Autodesk Inventor part; units mm, degrees
ref_plane "YZ Plane" through (0, 0, 0) normal (1, 0, 0) x (0, 1, 0)
ref_plane "XZ Plane" through (0, 0, 0) normal (0, 1, 0) x (-1, 0, 0)
ref_plane "XY Plane" through (0, 0, 0) normal (0, 0, 1) x (1, 0, 0)
sketch "草图1" plane through (0, 0, 0) normal (0, 0, 1) x (1, 0, 0)
  circle A0 centre (0, 0) radius 9.5
  dimension "d0" = 19
extrude "拉伸1" add sketch "草图1" along normal blind 4
sketch "草图2" plane through (0, 0, 0) normal (0, 0, -1) x (-1, 0, 0)
  circle A0 centre (0, 0) radius 9.5
  circle A1 centre (0, 0) radius 7
  dimension "d3" = 14
extrude "拉伸2" add sketch "草图2" along normal blind 3 contours A1
sketch "草图3" plane through (0, 0, -3) normal (0, 0, -1) x (-1, 0, 0)
  circle A0 centre (0, 0) radius 7
  circle A1 centre (0, 0) radius 8.3315
  dimension "d6" = 14
  dimension "d7" = 16.663
extrude "拉伸3" add sketch "草图3" along normal blind 7 contours A0 | A1
thread "螺纹1"
chamfer "倒角1" distance 1 angle 45 2 edges at (8.3315, 0, -10) (-9.5, 0, 4)
sketch "草图4" plane through (0, 0, 4) normal (0, 0, 1) x (1, 0, 0)
  circle A0 centre (0, 0) radius 8.5
  line L0 (0, 0) -> (0, 1)
  line L1 (0, 1) -> (21.5358, 1)
  line L2 (21.5358, 1) -> (-22.0631, 1)
  line L3 (-22.0631, 1) -> (-22.0631, -1)
  line L4 (-22.0631, -1) -> (21.5358, -1)
  line L5 (21.5358, -1) -> (21.5358, 1)
  dimension "d15" = 1
  dimension "d16" = 2
extrude "拉伸4" cut sketch "草图4" against normal blind 2 contours A0 L4 L2 L1 | A0 L1 L5 L4 | A0 L4 L3 L2
properties part number "螺塞" material "钢 AISI 1018 106 HR"
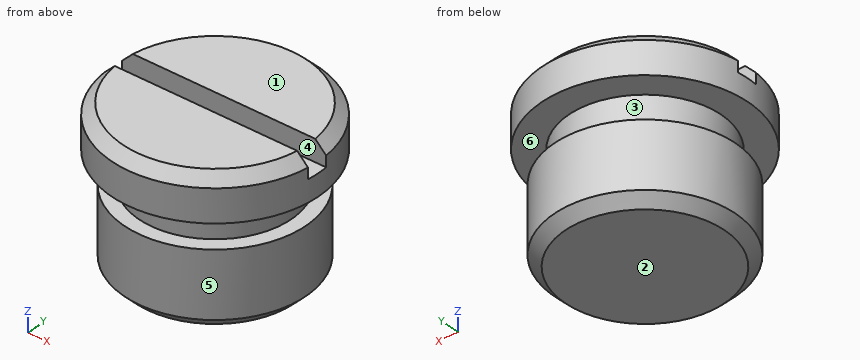
Design review of the part built by this model. Coordinates are the model's own, in mm. Face numbers are marked on the shaded views. A direction names the side the tool comes from. Give positions to 0.01 mm unless a question says otherwise; leave off trailing zeros. Loops run counter-clockwise (first coordinate to the right, second up) from the corner with the lowest first, then second, coordinate; pieces in that order, holes last. Notation, with made-up numbers: (67.5, 30) -> (121.5, 30) arc R29 cw to (121.5, 67) -> close; hole circle Ø3 at (-32.5, -11). An arc over 180 degrees is marked (long way). One line per question, with ' | ' between items. Start each with the question number.
(1) For the marked faces 4, 5 and 6, list the 3-axis set-ups (+Z, -Z, +X, -X, +Y, -Y) from which the entire face can be reached by the end or side of a thin tool; tool diameter is ignored.
(2) We need section B-B (y = 0). State the section outline as (x, z) points, and give its area (3 significant figures).
(3) We need section D-D (z = 1.25). State the section outline as (x, y) points.
(4) We need section C-C (z = -8.5). State the section outline as (x, y) points.
(5) For line 1 (Z direction, x = 0.25, y = -0.5); line 2 (Z direction, x = -3, y = -6.5); line 3 (Z direction, x = 6.75, y = 3.5), list the stretches that pass through material, from the lowest coordinate up.
(6) We need section A-A (x = 0). State the section outline as (y, z) points.
(7) Insertion check: P1, Ø2, axis at x = 4.5, z = -5.5, coming from the +Y side; P2, Ø8, axis at x = 4.5, z = -3, coming from the +Y side; P3, Ø3, axis at y = 5.5, z = -4.5, coming from the -X side. Each pin has a flat end and moves straight along its axis. Give the tip position at first contact, or say it passes through.
(8) Draft analysis for pull direction Z (two halves, no side actions). For the marked faces 1, 2 and 3, state which applies: +Z half, -Z half, draft (parallel to the pull), parting line (faces both ways), or undercut.
The answers:
1) face 4: +Z, +X, -X | face 5: -Z | face 6: none
2) outline: (-9.5, 0) -> (-7, 0) -> (-7, -3) -> (-8.33, -3) -> (-8.33, -9) -> (-7.33, -10) -> (7.33, -10) -> (8.33, -9) -> (8.33, -3) -> (7, -3) -> (7, 0) -> (9.5, 0) -> (9.5, 2) -> (-9.5, 2) -> close | area: 196 mm^2
3) outline: circle Ø19 at (0, 0)
4) outline: circle Ø16.66 at (0, 0)
5) line 1: z = -10 to 2 | line 2: z = -10 to -3, 0 to 4 | line 3: z = -9.73 to -3, 0 to 4
6) outline: (-9.5, 0) -> (-7, 0) -> (-7, -3) -> (-8.33, -3) -> (-8.33, -9) -> (-7.33, -10) -> (7.33, -10) -> (8.33, -9) -> (8.33, -3) -> (7, -3) -> (7, 0) -> (9.5, 0) -> (9.5, 3) -> (8.5, 4) -> (1, 4) -> (1, 2) -> (-1, 2) -> (-1, 4) -> (-8.5, 4) -> (-9.5, 3) -> close
7) P1: stops at y = 7.56 | P2: stops at y = 9.32 | P3: stops at x = -7.31
8) face 1: +Z half | face 2: -Z half | face 3: undercut
